Design review of the part built by this model. Coordinates are the model's own, in mm. A direction names the side the tool comes from. Give positions to 0.01 mm unless a question says otherwise; leave off trailing zeros. Loops run counter-clockwise (first coordinate to the right, second up) from the corner with the lowest first, then second, coordinate; pieces in that order, holes last. Notation, with made-up numbers: (14, -13) -> (33, -13) arc R31 cw to (33, 13) -> close; hole circle Ø8 at (86, 84). An arc over 180 degrees is marked (long way). Answer in a Markdown table with one row per item. Add a question column.
(1) Consider section B-B on x = 0. Count the separate pieces of the cut face and the enclosed holes in it, then the cut area to 3 significant figures.
(2) For line 1 (Z direction, x = 0, y = -3.25); line 2 (Z direction, x = 0, y = -4.75); line 3 (Z direction, x = 4.75, y = 1), list the stretches that pass through material, from the lowest coordinate up.
(3) Consider section A-A on z = -50. Write out the cut boundary in (x, y).
(4) For faces 1 (the cylindrical face through (0.481, -3.453, -73.474)), 2 (the cylindrical face through (2.285, 3.584, 3.451)), 3 (the flat face through (0, 3, -87)), 4 (the flat face through (2, 3, -9)), 5 (the cylindrical face through (1.517, -6.834, -59.059)), list the 3-axis set-ups (+Z, -Z, +X, -X, +Y, -Y) from which the entire face can be reached by the end or side of a thin tool; tool diameter is ignored.
(5) For pin 1 (2 mm diameter, centred on x = -0.5, y = 5.5, fed in from +Z); pin 2 (2 mm diameter, centred on x = 4.5, z = -36.5, fed in from +Y); pin 3 (7 mm diameter, centred on x = 0, z = -57, fed in from +Y), all flat-tipped, find the tip position at first contact; note any pin that passes through.
(6) Consider section D-D on z = -19. Write out the cut boundary in (x, y).
from build123d import *

# Parameters (mm, degrees)
SKETCH1_R               = 4.25
BOSS_EXTRUDE1_DEPTH     = 8
CHAMFER1_SIZE           = 1
SKETCH2_R               = 7
BOSS_EXTRUDE2_DEPTH     = 23.5
SKETCH4_R               = 11
BOSS_EXTRUDE3_DEPTH     = 4.5
SKETCH5_R               = 7
BOSS_EXTRUDE4_DEPTH     = 64
CUT_EXTRUDE2_DEPTH      = 94.305948363
CUT_EXTRUDE2_DEPTH_BACK = 94.305948363
SKETCH6_W               = 49
SKETCH6_H               = 7
CUT_EXTRUDE3_REACH      = 95.306
CUT_EXTRUDE3_END_RADIUS = 7
SKETCH7_R               = 1.6
CHAMFER2_SIZE           = 1
SKETCH8_W               = 4
SKETCH8_H               = 14
CUT_EXTRUDE4_DEPTH      = 10


with BuildPart() as part:
    # Sketch1 → Boss-Extrude1 (new body)
    with BuildSketch(Plane.XY):
        Circle(SKETCH1_R)
    extrude(amount=BOSS_EXTRUDE1_DEPTH)

    # Chamfer1
    chamfer1_edges = [part.edges().sort_by_distance(p)[0] for p in [
        (-4.25, 0, 8),
    ]]
    chamfer(chamfer1_edges, length=CHAMFER1_SIZE)

    # Sketch2 → Boss-Extrude2 (add)
    with BuildSketch(Plane(origin=(0, 0, 0), x_dir=(-1, 0, 0), z_dir=(0, 0, -1))):
        Circle(SKETCH2_R)
    extrude(amount=BOSS_EXTRUDE2_DEPTH)

    # Sketch4 → Boss-Extrude3 (add)
    with BuildSketch(Plane(origin=(0, 0, -23.5), x_dir=(-1, 0, 0), z_dir=(0, 0, -1))):
        Circle(SKETCH4_R)
    extrude(amount=BOSS_EXTRUDE3_DEPTH)

    # Sketch5 → Boss-Extrude4 (add)
    with BuildSketch(Plane(origin=(0, 0, -28), x_dir=(-1, 0, 0), z_dir=(0, 0, -1))):
        Circle(SKETCH5_R)
    extrude(amount=BOSS_EXTRUDE4_DEPTH)

    # Sketch6 → Cut-Extrude2 (cut, two sides: drawn at the far end of the back side and taken through both)
    with BuildSketch(Plane(origin=(0, 0, 0), x_dir=(0, 0, -1), z_dir=(1, 0, 0)).offset(-CUT_EXTRUDE2_DEPTH_BACK)):
        with Locations((62.5, 3.5)):
            Rectangle(SKETCH6_W, SKETCH6_H)
    extrude(amount=CUT_EXTRUDE2_DEPTH + CUT_EXTRUDE2_DEPTH_BACK, mode=Mode.SUBTRACT)

    # Cut-Extrude3: up to this cylinder (the profile starts inside it)
    cut_extrude3_end = Plane(origin=(0, 0, -62.5), z_dir=(0, 0, 1)) * Cylinder(CUT_EXTRUDE3_END_RADIUS, 230.612, mode=Mode.PRIVATE)
    # Sketch7 → Cut-Extrude3 (cut, up to the surface)
    with BuildSketch(Plane(origin=(0, 0, 0), x_dir=(1, 0, 0), z_dir=(0, 1, 0)), mode=Mode.PRIVATE) as cut_extrude3_sk1:
        with Locations(Location((0, 75, 0), (0, 0, 270))):
            Circle(SKETCH7_R)
    cut_extrude3_tool1 = extrude(cut_extrude3_sk1.sketch, amount=-CUT_EXTRUDE3_REACH, mode=Mode.PRIVATE) & cut_extrude3_end
    add(cut_extrude3_tool1.solids().sort_by_distance((0, 0, -75))[0], mode=Mode.SUBTRACT)
    # Sketch7 → Cut-Extrude3 (cut, up to the surface)
    with BuildSketch(Plane(origin=(0, 0, 0), x_dir=(1, 0, 0), z_dir=(0, 1, 0)), mode=Mode.PRIVATE) as cut_extrude3_sk2:
        with Locations(Location((0, 50, 0), (0, 0, 270))):
            Circle(SKETCH7_R)
    cut_extrude3_tool2 = extrude(cut_extrude3_sk2.sketch, amount=-CUT_EXTRUDE3_REACH, mode=Mode.PRIVATE) & cut_extrude3_end
    add(cut_extrude3_tool2.solids().sort_by_distance((0, 0, -50))[0], mode=Mode.SUBTRACT)

    # Chamfer2
    chamfer2_edges = [part.edges().sort_by_distance(p)[0] for p in [
        (7, 0, -92),
    ]]
    chamfer(chamfer2_edges, length=CHAMFER2_SIZE)

    # Sketch8 → Cut-Extrude4 (cut)
    with BuildSketch(Plane(origin=(0, 0, 0), x_dir=(1, 0, 0), z_dir=(0, 1, 0))):
        with Locations((0, 9)):
            Rectangle(SKETCH8_W, SKETCH8_H)
    extrude(amount=CUT_EXTRUDE4_DEPTH, mode=Mode.SUBTRACT)


solid = part.part
Values follow:
| question | item | result |
|---|---|---|
| 1 | separate pieces | 3 |
| 1 | enclosed holes | 0 |
| 1 | area | 904 mm2 |
| 2 | line 1 | -92 to -76.6, -73.4 to -51.6, -48.4 to 8 |
| 2 | line 2 | -92 to -76.6, -73.4 to -51.6, -48.4 to 0 |
| 2 | line 3 | -92 to -87, -38 to 0 |
| 3 | outline | (-7, 0) arc R7 ccw to (-1.6, -6.81) -> (-1.6, 0) -> close; (1.6, -6.81) arc R7 ccw to (7, 0) -> (1.6, 0) -> close |
| 4 | face 1 | +Y, -Y |
| 4 | face 2 | +Z |
| 4 | face 3 | +X, -X, +Y |
| 4 | face 4 | +Y |
| 4 | face 5 | -Z |
| 5 | pin 1 | z = 0 |
| 5 | pin 2 | y = 6.06 |
| 5 | pin 3 | y = 0 |
| 6 | outline | circle Ø14 at (0, 0) |
